Check sheet for the modelled part. Datum: model origin and axes. Units: mm. Coordinates: 2 decimals unless noted, no trailing zeros. Loops run counter-clockwise (first coordinate to the right, second up) from the corner with the lowest first, then second, coordinate; pieces in that order, holes last. Notation, with made-up numbers: M 65.5,-33.5 L 116.5,-33.5 A22 ccw 116.5,-1.5 Z; hole C 18,-10 d9. An arc over 180 degrees is marked long. Return JSON: item names as keys, results as strings.
Autodesk Inventor part; units mm, degrees
ref_plane "YZ Plane" through (0, 0, 0) normal (1, 0, 0) x (0, 1, 0)
ref_plane "XZ Plane" through (0, 0, 0) normal (0, 1, 0) x (-1, 0, 0)
ref_plane "XY Plane" through (0, 0, 0) normal (0, 0, 1) x (1, 0, 0)
sketch "スケッチ1" plane through (0, 0, 0) normal (0, 0, 1) x (1, 0, 0)
  line L0 (0, 0) -> (10, 0)
  line L1 (10, 0) -> (10, 285)
  line L2 (10, 285) -> (0, 285)
  line L3 (0, 285) -> (0, 0)
  dimension "d0" = 10
  dimension "d1" = 285
extrude "押し出し1" add sketch "スケッチ1" along normal blind 10
sketch "スケッチ2" plane through (10, 0, 0) normal (1, 0, 0) x (0, 0, -1)
  line L0 (0, 0) -> (-10, 0)
  line L1 (0, 285) -> (-10, 285)
  point P0 (-5, 5)
  point P1 (-5, 0)
  point P2 (-5, 0)
  point P3 (-5, 0)
  point P4 (-5, 285)
  dimension "d4" = 5
hole "穴1" at (10, 5, 5) direction (-1, 0, 0) diameter 3.1 end through all
sketch "スケッチ3" plane through (0, 0, 10) normal (0, 0, 1) x (1, 0, 0)
  line L0 (0, 0) -> (10, 0)
  line L1 (10, 285) -> (0, 285)
  point P0 (5, 15)
  point P1 (5, 280)
  point P2 (5, 0)
  point P3 (5, 0)
  point P4 (5, 0)
  point P5 (5, 285)
  dimension "d13" = 15
  dimension "d14" = 5
hole "穴2" at (5, 15, 10) at (5, 280, 10) direction (0, 0, -1) diameter 3.1 end through all
properties part number "Tate"
1) Go/stop test with a flat-tipped pin: pin 1 Ø1.9 at (y, z) = (5, 5) entering from +X. Record where the tip stops, or that it passes through.
Answers:
{"pin 1": "through"}
2) Section check B-B on x = 5. Record the cut outline in (y, z), then the cut area to 3 significant figures.
Answers:
{"outline": "M 0,0 L 13.45,0 L 13.45,10 L 0,10 Z; M 16.55,0 L 278.45,0 L 278.45,10 L 16.55,10 Z; M 281.55,0 L 285,0 L 285,10 L 281.55,10 Z; hole C 5,5 d3.1", "area": "2,780 mm²"}
3) Section check A-A on z = 5. Record the cut outline in (x, y), then the cut area to 3 significant figures.
Answers:
{"outline": "M 0,0 L 10,0 L 10,3.45 L 0,3.45 Z; M 0,6.55 L 10,6.55 L 10,285 L 0,285 Z; hole C 5,15 d3.1; hole C 5,280 d3.1", "area": "2,800 mm²"}
4) Scan lines: line 1 along Y through (x, z) = (5, 2.75); line 2 along X through (y, z) = (15, 4.25); line 3 along Y through (x, z) = (2.75, 5). Record each from-to range of solid material in increasing order. Write a range as [from, to].
Answers:
{"line 1": "[0, 13.45], [16.55, 278.45], [281.55, 285]", "line 2": "[0, 3.45], [6.55, 10]", "line 3": "[0, 3.45], [6.55, 285]"}
